from build123d import *

# Parameters (mm, degrees)
ESQUISSE1_W             = 61.5
ESQUISSE1_H             = 43.75
BOSS_EXTRU_1_DEPTH      = 77
ENL_V_MAT_EXTRU_4_REACH = 79
ESQUISSE3_W             = 9.3
ESQUISSE3_H             = 11
ESQUISSE3_W_2           = 12
ESQUISSE3_H_2           = 10.6
ESQUISSE6_W             = 53.5
ESQUISSE6_H             = 35.75
ENL_V_MAT_EXTRU_5_DEPTH = 73
CONG_4_R                = 2


with BuildPart() as part:
    # Esquisse1 → Boss.-Extru.1 (new body)
    with BuildSketch(Plane.XY):
        with Locations((-0.850502513, 12.751256281)):
            Rectangle(ESQUISSE1_W, ESQUISSE1_H)
    extrude(amount=BOSS_EXTRU_1_DEPTH)

    # Esquisse3 → Enlèv. mat.-Extru.4 (cut, up to next)
    with BuildSketch(Plane.XY.offset(77), mode=Mode.PRIVATE) as enl_v_mat_extru_4_sk1:
        with Locations((17.819497487, 5.476256281)):
            Rectangle(ESQUISSE3_W, ESQUISSE3_H)
    enl_v_mat_extru_4_tool1 = extrude(enl_v_mat_extru_4_sk1.sketch, amount=-ENL_V_MAT_EXTRU_4_REACH, mode=Mode.PRIVATE) & part.part
    add(enl_v_mat_extru_4_tool1.solids().sort_by_distance((17.819497, 5.476256, 77))[0], mode=Mode.SUBTRACT)
    # Esquisse3 → Enlèv. mat.-Extru.4 (cut, up to next)
    with BuildSketch(Plane.XY.offset(77), mode=Mode.PRIVATE) as enl_v_mat_extru_4_sk2:
        with Locations((-9.900502513, 5.576256281)):
            Rectangle(ESQUISSE3_W_2, ESQUISSE3_H_2)
    enl_v_mat_extru_4_tool2 = extrude(enl_v_mat_extru_4_sk2.sketch, amount=-ENL_V_MAT_EXTRU_4_REACH, mode=Mode.PRIVATE) & part.part
    add(enl_v_mat_extru_4_tool2.solids().sort_by_distance((-9.900503, 5.576256, 77))[0], mode=Mode.SUBTRACT)

    # Esquisse6 → Enlèv. mat.-Extru.5 (cut)
    with BuildSketch(Plane(origin=(0, 0, 0), x_dir=(-1, 0, 0), z_dir=(0, 0, -1))):
        with Locations((0.850502513, 12.751256281)):
            Rectangle(ESQUISSE6_W, ESQUISSE6_H)
    extrude(amount=-ENL_V_MAT_EXTRU_5_DEPTH, mode=Mode.SUBTRACT)

    # Congé4
    cong_4_edges = [part.edges().sort_by_distance(p)[0] for p in [
        (29.899497487, 12.751256281, 77),
        (-0.850502513, 34.626256281, 77),
        (-31.600502513, 12.751256281, 77),
        (-31.600502513, 34.626256281, 38.5),
        (29.899497487, 34.626256281, 38.5),
        (29.899497487, -9.123743719, 38.5),
        (-31.600502513, -9.123743719, 38.5),
        (-0.850502513, -9.123743719, 77),
    ]]
    fillet(cong_4_edges, radius=CONG_4_R)


solid = part.part
CAD build for the part. Positions are in the model's coordinates, mm. A direction names the side the tool comes from. Give positions to 0.01 mm unless a question says otherwise; leave off trailing zeros. Write each loop counter-clockwise with the first axis right and the second up, starting at its lowest first coordinate (ties: lowest second). Pieces come first, ordered by that corner, then holes. Notation, with made-up numbers: M 44.5,19 L 61.5,19 A12 cw 61.5,42 Z; hole C 80.25,10.5 d2. An arc over 180 degrees is marked long. Put each result on its own line as item: value. Start each with the question number.
(1) Flat gauge pin, fed straight in: pin 1 Ø8 at (x, y) = (-15.5, 21.5) entering from -Z. Where does the tip first touch, or does it go through?
(2) Band-saw the part on D-D, the plane x = 6. Write the cut outline in (y, z).
(3) Which spindle directions (+Z, -Z, +X, -X, +Y, -Y) get a long thin tool onto all of the face, cutting with end or side? Do faces 4 (the face through (-1, -6, 0)), 5 (the face through (0, -5.124, 36)), 6 (the face through (-3.901, 6, 75)). Say none if no direction does.
(4) Probe L1, parallel to X at y = 24.5, z = 68; L2, parallel to Y at x = -1, z = 15; L3, parallel to Z at x = 11, y = -2. List the from-to ranges inside material, lowest first.
(5) Band-saw the part on B-B, the plane x = -11.5. Write the cut outline in (y, z).
(6) Band-saw the part on C-C, the plane z = 59. Write the cut outline in (x, y), and give its area (3 significant figures).
(7) Band-saw the part on A-A, the plane y = 10. Write the cut outline in (x, z).
(8) Mould opens along X. For faces 1 (the face through (29.298, 34.056, 38.025)), 2 (the face through (25.899, 13, 36)), 3 (the face through (-31.03, -8.52, 38.02)) say: +X half, -X half, draft (parallel to the pull), parting line (faces both ways), or undercut.
Response values:
1. pin 1: stops at z = 73
2. outline: M -9.12,0 L -5.12,0 L -5.12,73 L 30.63,73 L 30.63,0 L 34.63,0 L 34.63,75 A2 ccw 32.63,77 L -7.12,77 A2 ccw -9.12,75 Z
3. face 4: -Z, +X, -X, +Y, -Y
3. face 5: -Z
3. face 6: +Z, -Z
4. L1: x = -31.6 to -27.6, 25.9 to 29.9
4. L2: y = -9.12 to -5.12, 30.63 to 34.63
4. L3: z = 73 to 77
5. outline: M -9.12,0 L -5.12,0 L -5.12,73 L 0.28,73 L 0.28,77 L -7.12,77 A2 ccw -9.12,75 Z; M 10.88,73 L 30.63,73 L 30.63,0 L 34.63,0 L 34.63,75 A2 ccw 32.63,77 L 10.88,77 Z
6. outline: M -31.6,-7.12 A2 ccw -29.6,-9.12 L 27.9,-9.12 A2 ccw 29.9,-7.12 L 29.9,32.63 A2 ccw 27.9,34.63 L -29.6,34.63 A2 ccw -31.6,32.63 Z; hole M -27.6,-5.12 L 25.9,-5.12 L 25.9,30.63 L -27.6,30.63 Z
6. area: 775 mm2
7. outline: M -31.6,0 L -27.6,0 L -27.6,73 L -15.9,73 L -15.9,77 L -29.6,77 A2 ccw -31.6,75 Z; M -3.9,73 L 13.17,73 L 13.17,77 L -3.9,77 Z; M 22.47,73 L 25.9,73 L 25.9,0 L 29.9,0 L 29.9,75 A2 ccw 27.9,77 L 22.47,77 Z
8. face 1: +X half
8. face 2: undercut
8. face 3: -X half
